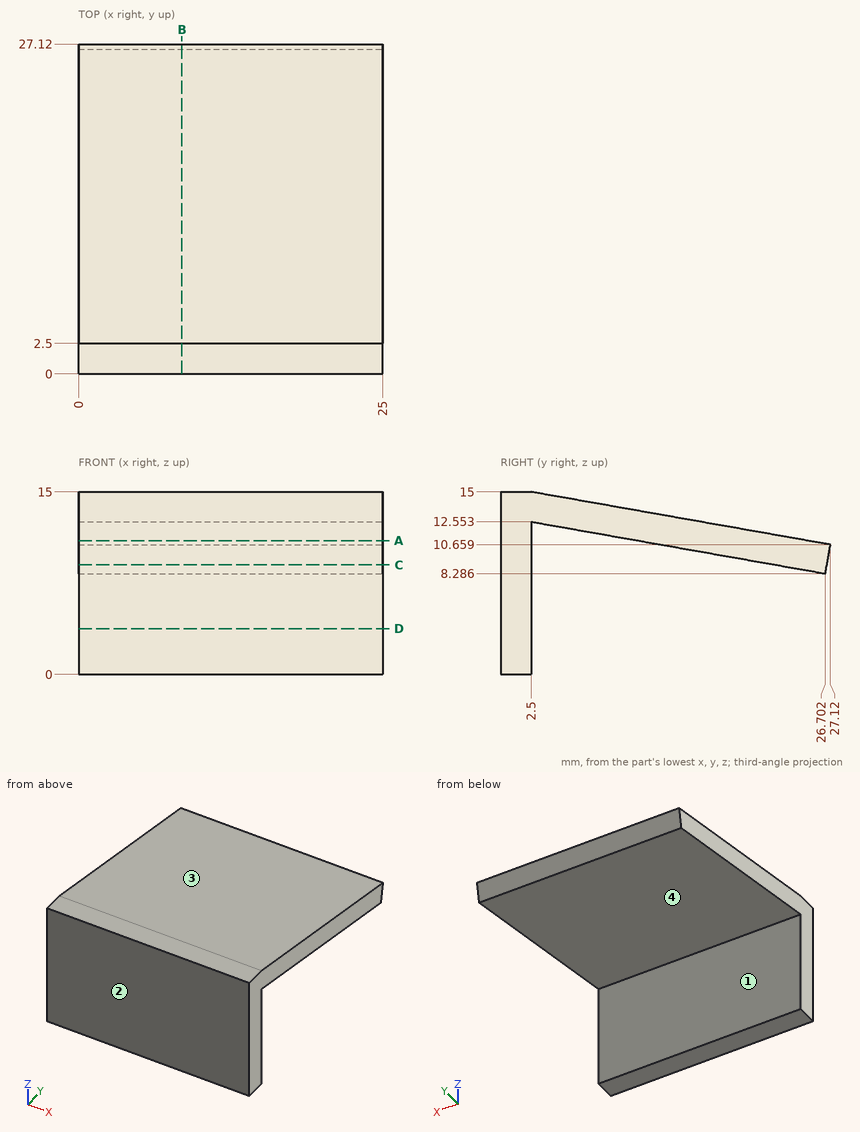
Verification items for this drawing (mm, ordinates from the low corner). Coordinates: 2 decimals unless noted, no trailing zeros. Order: outer loops, then holes, each group sorted by start corner. A loop starts at its lowest first (then second) coordinate and runs counter-clockwise, first axis right, second up. Notation, with made-up numbers: (82, -24.5) -> (95, -24.5) arc R4 cw to (95, -19.5) -> close; hole circle Ø2 at (50.5, 73). An arc over 180 degrees is marked (long way). Put each result on its own line as item: value. Start each with the question number.
1. Go/stop test with flat-tipped pins: pin 1 Ø1 at (x, z) = (16.5, 7.5) entering from +Y; pin 2 Ø2 at (x, y) = (21.5, 11.5) entering from +Z; pin 3 Ø5 at (x, y) = (18, 20.5) entering from +Z. Record where each tip stops, or that it passes through.
2. Cross-section at B-B, the plane x = 8.5. Record the boundary of the cut face in (y, z) (1 decimal).
3. Cross-section at D-D, the plane z = 3.75. Record the boundary of the cut face in (x, y).
4. Material ranges on L1, parallel to Y at x = 13.25, z = 6.75; L2, parallel to Z at x = 1.25, y = 15 (1 decimal); L3, parallel to Z at x = 7, y = 24.5, recorded low to high. Write a range as [from, to].
5. Cross-section at C-C, the plane z = 9. Record the boundary of the cut face in (x, y).
6. Cross-section at A-A, the plane z = 11. Record the boundary of the cut face in (x, y) (1 decimal).
7. Mould release check, pull along Y, two halves, no side actions. Record for the marked faces 1, 2, 3 and 4: released by +Y, released by -Y, zero draft, split by the parting line, or undercut.
Computed:
1. pin 1: y = 2.5
1. pin 2: z = 13.59
1. pin 3: z = 12.27
2. outline: (0, 0) -> (2.5, 0) -> (2.5, 12.6) -> (26.7, 8.3) -> (27.1, 10.7) -> (2.5, 15) -> (0, 15) -> close
3. outline: (0, 0) -> (25, 0) -> (25, 2.5) -> (0, 2.5) -> close
4. L1: [0, 2.5]
4. L2: [10.3, 12.8]
4. L3: [8.67, 11.12]
5. outline: (0, 0) -> (25, 0) -> (25, 2.5) -> (0, 2.5) -> close; (0, 22.65) -> (25, 22.65) -> (25, 26.83) -> (0, 26.83) -> close
6. outline: (0, 0) -> (25, 0) -> (25, 2.5) -> (0, 2.5) -> close; (0, 11.3) -> (25, 11.3) -> (25, 25.2) -> (0, 25.2) -> close
7. face 1: undercut
7. face 2: released by -Y
7. face 3: released by +Y
7. face 4: undercut
